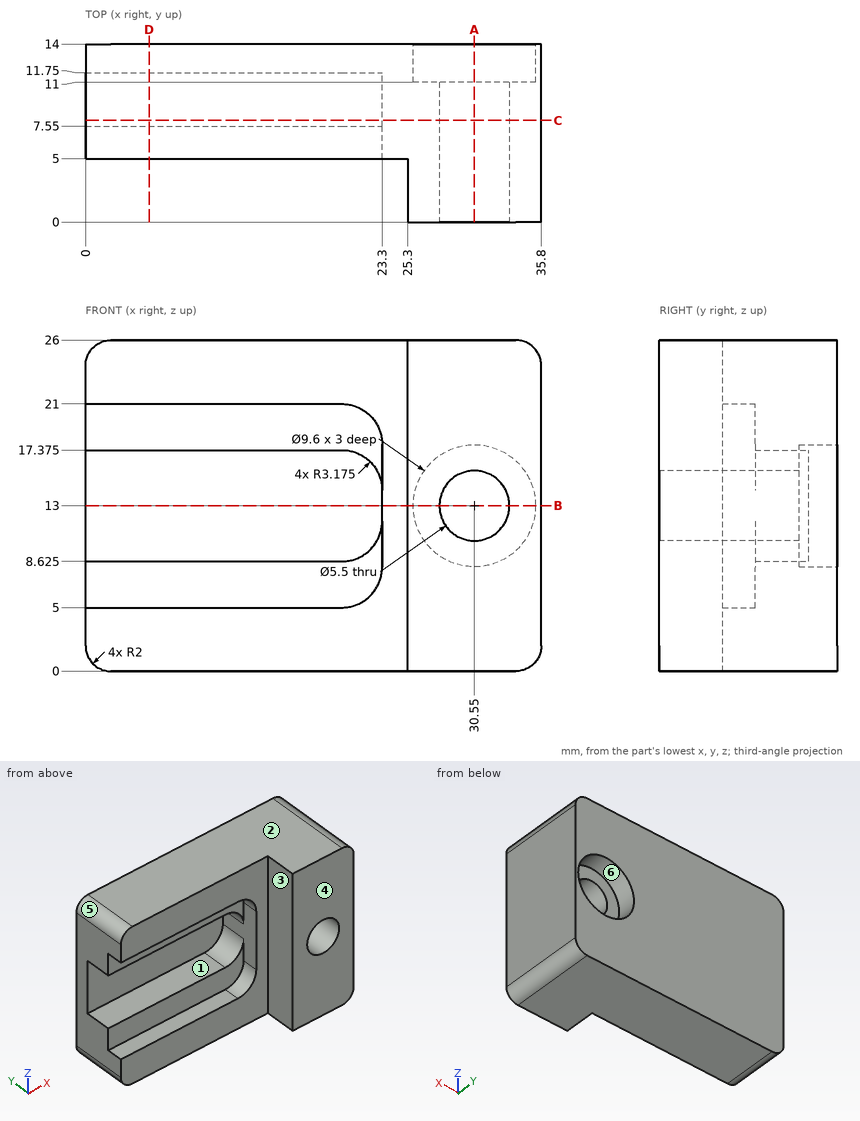
Here's the drawing with two shaded views (mm, measured from the low corner). I have some questions. A direction names the side the tool comes from. Round coordinates to 2 decimals unless told otherwise and drop trailing zeros. Loops run counter-clockwise (first coordinate to the right, second up) from the corner with the lowest first, then second, coordinate; pieces in that order, holes last. Notation, with made-up numbers: M -7,6.25 L 22,6.25 A23 ccw 22,35.25 Z; hole C 46,62 d1. An arc over 180 degrees is marked long. Put each result on its own line as item: value.
Q1. Imagine slicing it at C-C (y = 8). Write out the boundary of the cut face in (x, z) (3 decimals), then the cut area to 3 significant figures.
Check result:
outline: M 0,2 A2 ccw 2,0 L 33.8,0 A2 ccw 35.8,2 L 35.8,24 A2 ccw 33.8,26 L 2,26 A2 ccw 0,24 L 0,17.375 L 20.125,17.375 A3.175 cw 23.3,14.2 L 23.3,11.8 A3.175 cw 20.125,8.625 L 0,8.625 Z; hole C 30.55,13 d5.5
area: 704 mm2
Q2. Imagine slicing it at A-A (x = 30.55). Write out the boundary of the cut face in (y, z), then the cut area to 3 significant figures.
Check result:
outline: M 0,0 L 14,0 L 14,8.2 L 11,8.2 L 11,10.25 L 0,10.25 Z; M 0,15.75 L 11,15.75 L 11,17.8 L 14,17.8 L 14,26 L 0,26 Z
area: 275 mm2
Q3. For pin 1 (2.5 mm diameter, centred on x = 10.5, z = 11, fed in from -Y); pin 2 (7 mm diameter, centred on x = 30.55, z = 13, fed in from +Y); pin 3 (2 mm diameter, centred on y = 8, z = 12.5, fed in from -X), each with a flat end and sliding along its axis, tell me the tip position at first contact or that it passes through.
Check result:
pin 1: y = 11.75
pin 2: y = 11
pin 3: x = 23.29
Q4. Thinking about a two-plate mould opening in X: for the marked faces 4, 5 and 6, which applies, released by +X, released by -X, zero draft, split by the parting line, or undercut?
Check result:
face 4: zero draft
face 5: released by -X
face 6: undercut
Q5. On a 3-axis mill with a long thin cutter (end or side, diameter ignored), from which of +Z, -Z, +X, -X, +Y, -Y can I reach the whole of each face in a straight line? I mean the marked faces 1, 2 and 3. Say none if no direction works.
Check result:
face 1: -X, -Y
face 2: +Z, +X, -X, +Y, -Y
face 3: +Z, -Z, -X, -Y
Q6. I need wall thicknesses on probe 1 along Z at (x, y) = (11.5, 8.75) (3 decimals); probe 2 along Z at (x, y) = (30.55, 11.9); probe 3 along X at (y, z) = (4.5, 13). Which ranges of each line are inside material? Lowest first, please.
Check result:
probe 1: 0 to 8.625, 17.375 to 26
probe 2: 0 to 8.2, 17.8 to 26
probe 3: 25.3 to 27.8, 33.3 to 35.8
Q7. Imagine slicing it at B-B (z = 13). Write out the boundary of the cut face in (x, y), then the cut area to 3 significant figures.
Check result:
outline: M 0,11.75 L 23.3,11.75 L 23.3,5 L 25.3,5 L 25.3,0 L 27.8,0 L 27.8,11 L 25.75,11 L 25.75,14 L 0,14 Z; M 33.3,0 L 35.8,0 L 35.8,14 L 35.35,14 L 35.35,11 L 33.3,11 Z
area: 128 mm2
Q8. Imagine slicing it at D-D (x = 5). Write out the boundary of the cut face in (y, z) (3 decimals).
Check result:
outline: M 5,0 L 14,0 L 14,26 L 5,26 L 5,21 L 7.55,21 L 7.55,17.375 L 11.75,17.375 L 11.75,8.625 L 7.55,8.625 L 7.55,5 L 5,5 Z
